Drawing for the job (mm, zero at the part's lowest x, y, z). A direction names the side the tool comes from. Round coordinates to 2 decimals unless told otherwise and drop trailing zeros. Write each loop counter-clockwise with the first axis right and the second up, starting at its lowest first coordinate (ties: lowest second). Pieces come first, ordered by that corner, then holes. Notation, with made-up numbers: M 47.25,9.25 L 83.25,9.25 A22 ccw 83.25,42.25 Z; hole C 4,87 d7. An arc over 180 degrees is marked long. Use a Markdown table: item, result.
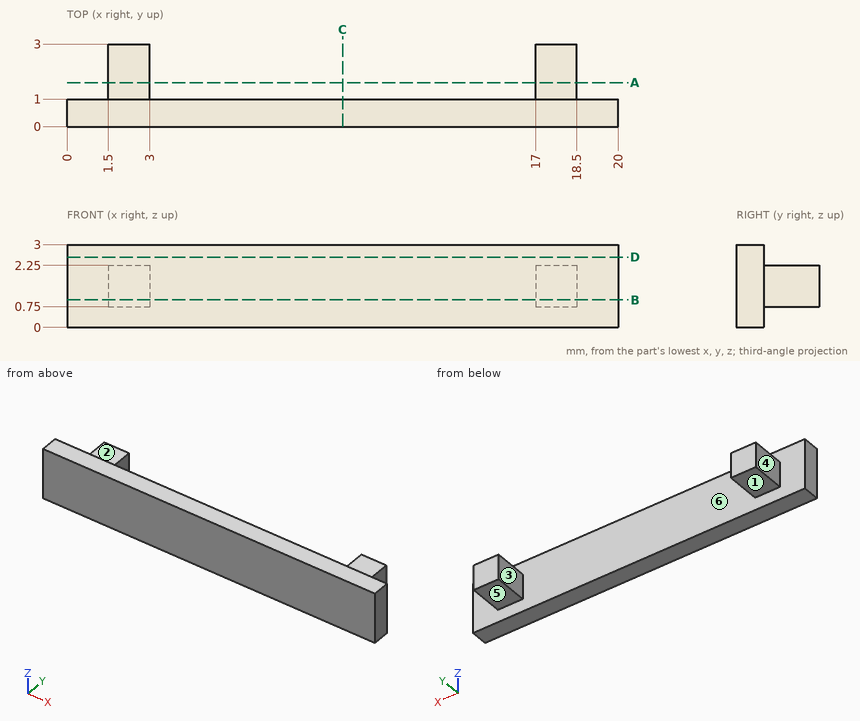
Q1. Cut at C-C on x = 10. Give the cut face in (y, z), and give its area (3 significant figures).
Response values:
| item | result |
|---|---|
| outline | M 0,0 L 1,0 L 1,3 L 0,3 Z |
| area | 3.00 mm2 |
Q2. Cut at A-A on y = 1.6. Give the cut face in (x, z), and give its area (3 significant figures).
Response values:
| item | result |
|---|---|
| outline | M 1.5,0.75 L 3,0.75 L 3,2.25 L 1.5,2.25 Z; M 17,0.75 L 18.5,0.75 L 18.5,2.25 L 17,2.25 Z |
| area | 4.50 mm2 |
Q3. Two-plate mould, pull along X, no slides. Class the marked faces 4, 5 and 6: +X half, -X half, draft (parallel to the pull), parting line (faces both ways), or undercut.
Response values:
| item | result |
|---|---|
| face 4 | -X half |
| face 5 | draft |
| face 6 | undercut |
Q4. Drill centre lines: L1, parallel to X at y = 2.85, z = 1.05; L2, parallel to Y at x = 17.25, z = 2.5; L3, parallel to Z at x = 2.25, y = 1.8. Where is each one in solid material? Low to high.
Response values:
| item | result |
|---|---|
| L1 | x = 1.5 to 3, 17 to 18.5 |
| L2 | y = 0 to 1 |
| L3 | z = 0.75 to 2.25 |
Q5. Which spindle directions (+Z, -Z, +X, -X, +Y, -Y) get a long thin tool onto all of the face, cutting with end or side? Do the marked faces 1, 2 and 3. Say none if no direction does.
Response values:
| item | result |
|---|---|
| face 1 | -Z, +X, -X, +Y |
| face 2 | +Z, +X, -X, +Y |
| face 3 | +Z, -Z, +Y |
Q6. Cut at B-B on z = 1. Give the cut face in (x, y).
Response values:
| item | result |
|---|---|
| outline | M 0,0 L 20,0 L 20,1 L 18.5,1 L 18.5,3 L 17,3 L 17,1 L 3,1 L 3,3 L 1.5,3 L 1.5,1 L 0,1 Z |
Q7. Drop flat-ended pins along their axis: P1, Ø0.8, axis at x = 2, y = 2, coming from the -Z side; P2, Ø1.6, axis at y = 2, z = 1.5, coming from the +X side; P3, Ø1.2, axis at y = 2, z = 1.5, coming from the -X side. Give the stop position or say it passes through.
Response values:
| item | result |
|---|---|
| P1 | stops at z = 0.75 |
| P2 | stops at x = 18.5 |
| P3 | stops at x = 1.5 |
Q8. Cut at D-D on z = 2.55. Give the cut face in (x, y).
Response values:
| item | result |
|---|---|
| outline | M 0,0 L 20,0 L 20,1 L 0,1 Z |
